Input: part model. Units: mm. Frame: model coordinates. A direction names the side the tool comes from. Give positions to 0.01 mm unless a question says otherwise; leave off trailing zeros. Loops run counter-clockwise (first coordinate to the right, second up) from the corner with the lowest first, then second, coordinate; pieces in that order, holes last. Notation, with made-up numbers: (34, 37.25) - (82, 37.25) arc R19 cw to (82, 62.25) - close; hole circle Ø1 at (6.5, -4.5). An arc over 180 degrees is marked (long way). Answer as a JSON object with one key per item and string values.
from build123d import *

# Parameters (mm, degrees)
SKETCH_1_R               = 5
EXTRUDE_1_DEPTH          = 18.5
SKETCH_2_R               = 6
EXTRUDE_2_DEPTH          = 4
SKETCH_3_R               = 5
EXTRUDE_3_DEPTH          = 10
SKETCH_5_R               = 3.1
CUT_EXTRUDE_2_DEPTH      = 25
CUT_EXTRUDE_3_DEPTH      = 34.589432862
CUT_EXTRUDE_3_DEPTH_BACK = 34.589432862
SKETCH_6_R               = 2.1
SKETCH_7_R               = 4
EXTRUDE_4_DEPTH          = 8.5
SKETCH_4_R               = 1.6
CUT_EXTRUDE_1_DEPTH      = 42.868842831


with BuildPart() as part:
    # ｽｹｯﾁ1 → ﾎﾞｽ - 押し出し1 (new body)
    with BuildSketch(Plane.XY):
        Circle(SKETCH_1_R)
    extrude(amount=EXTRUDE_1_DEPTH)

    # ｽｹｯﾁ2 → ﾎﾞｽ - 押し出し2 (add)
    with BuildSketch(Plane.XY.offset(18.5)):
        Circle(SKETCH_2_R)
    extrude(amount=EXTRUDE_2_DEPTH)

    # ｽｹｯﾁ3 → ﾎﾞｽ - 押し出し3 (add)
    with BuildSketch(Plane.XY.offset(22.5)):
        Circle(SKETCH_3_R)
    extrude(amount=EXTRUDE_3_DEPTH)

    # ｽｹｯﾁ5 → ｶｯﾄ - 押し出し2 (cut)
    with BuildSketch(Plane.XY.offset(32.5)):
        Circle(SKETCH_5_R)
    extrude(amount=-CUT_EXTRUDE_2_DEPTH, mode=Mode.SUBTRACT)

    # ｽｹｯﾁ6 → ｶｯﾄ - 押し出し3 (cut, two sides: drawn at the far end of the back side and taken through both)
    with BuildSketch(Plane(origin=(0, 0, 0), x_dir=(0, 0, -1), z_dir=(1, 0, 0)).offset(-CUT_EXTRUDE_3_DEPTH_BACK)):
        with Locations((-11, 0)):
            Circle(SKETCH_6_R)
    extrude(amount=CUT_EXTRUDE_3_DEPTH + CUT_EXTRUDE_3_DEPTH_BACK, mode=Mode.SUBTRACT)

    # ｽｹｯﾁ7 → ﾎﾞｽ - 押し出し4 (add)
    with BuildSketch(Plane(origin=(0, 0, 0), x_dir=(-1, 0, 0), z_dir=(0, 0, -1))):
        Circle(SKETCH_7_R)
    extrude(amount=EXTRUDE_4_DEPTH)

    # ｽｹｯﾁ4 → ｶｯﾄ - 押し出し1 (cut, through all)
    with BuildSketch(Plane.XY.offset(32.5)):
        Circle(SKETCH_4_R)
    extrude(amount=-CUT_EXTRUDE_1_DEPTH, mode=Mode.SUBTRACT)


solid = part.part
Item 1: Cut plane A-A (x = 0). Return loops of the section in (y, z), then the cut area to 3 significant figures.
Geometry check:
{"outline": "(-6, 18.5) - (-5, 18.5) - (-5, 0) - (-4, 0) - (-4, -8.5) - (-1.6, -8.5) - (-1.6, 7.5) - (-3.1, 7.5) - (-3.1, 32.5) - (-5, 32.5) - (-5, 22.5) - (-6, 22.5) - close; (1.6, -8.5) - (4, -8.5) - (4, 0) - (5, 0) - (5, 18.5) - (6, 18.5) - (6, 22.5) - (5, 22.5) - (5, 32.5) - (3.1, 32.5) - (3.1, 7.5) - (1.6, 7.5) - close", "area": "195 mm2"}
Item 2: Contact query for flat-ended pins moving along their axis: P1, Ø3, axis at x = -4, z = -0.5, coming from the -Y side; P2, Ø3.5, axis at x = 0, y = 0, coming from the -Z side; P3, Ø3, axis at x = 1.5, z = 12.5, coming from the -Y side; P4, Ø1.5, axis at y = -4.5, z = 10.5, coming from the -X side. Output: stop coordinate, or through.
Geometry check:
{"P1": "stops at y = -4.28", "P2": "stops at z = -8.5", "P3": "stops at y = -5", "P4": "stops at x = -3.31"}
Item 3: Material intervals for line 1 (Y direction, x = 0, z = 27.5); line 2 (Z direction, x = -1.75, y = 2.25), sorted ascending. Write a range as [from, to].
Geometry check:
{"line 1": "y = [-5, -3.1], [3.1, 5]", "line 2": "z = [-8.5, 7.5]"}
Item 4: Access query for faces 1 (the face through (-0.1, -3.3, 32.5)), 2 (the face through (2.957, 0.931, 20.175)), 3 (the face through (0.867, -3.905, -4.19)). Directions: +Z, -Z, +X, -X, +Y, -Y. A direction counts if a zero-diameter tool reaches every point of the face in a straight line with its end or side. Return the directions, or none.
Geometry check:
{"face 1": "+Z, +X, -X, +Y, -Y", "face 2": "+Z", "face 3": "-Z"}
Item 5: Cut plane B-B (y = 0). Give the number of separate pieces and of enclosed holes in the cut face, then the cut area to 3 significant figures.
Geometry check:
{"separate pieces": "4", "enclosed holes": "0", "area": "179 mm2"}
Item 6: Cut plane D-D (z = 3). Return loops of the section in (x, y), then the cut area to 3 significant figures.
Geometry check:
{"outline": "circle Ø10 at (0, 0); hole circle Ø3.2 at (0, 0)", "area": "70.5 mm2"}
Item 7: Cut plane C-C (z = 11). Return loops of the section in (x, y), then the cut area to 3 significant figures.
Geometry check:
{"outline": "(-4.54, -2.1) arc R5 ccw to (4.54, -2.1) - (2.28, -2.1) arc R3.1 cw to (-2.28, -2.1) - close; (-4.54, 2.1) - (-2.28, 2.1) arc R3.1 cw to (2.28, 2.1) - (4.54, 2.1) arc R5 ccw to start", "area": "31.5 mm2"}
Item 8: Mould query, pull axis Y, two halves, no side actions, for faces 4 (the face through (1.3, -1.3, 7.5)), 5 (the face through (4.77, 1.5, 9.12)), 6 (the face through (-4, 4, 22.5)). Classes: released by +Y, released by -Y, zero draft, split by the parting line, or undercut.
Geometry check:
{"face 4": "undercut", "face 5": "split by the parting line", "face 6": "zero draft"}
